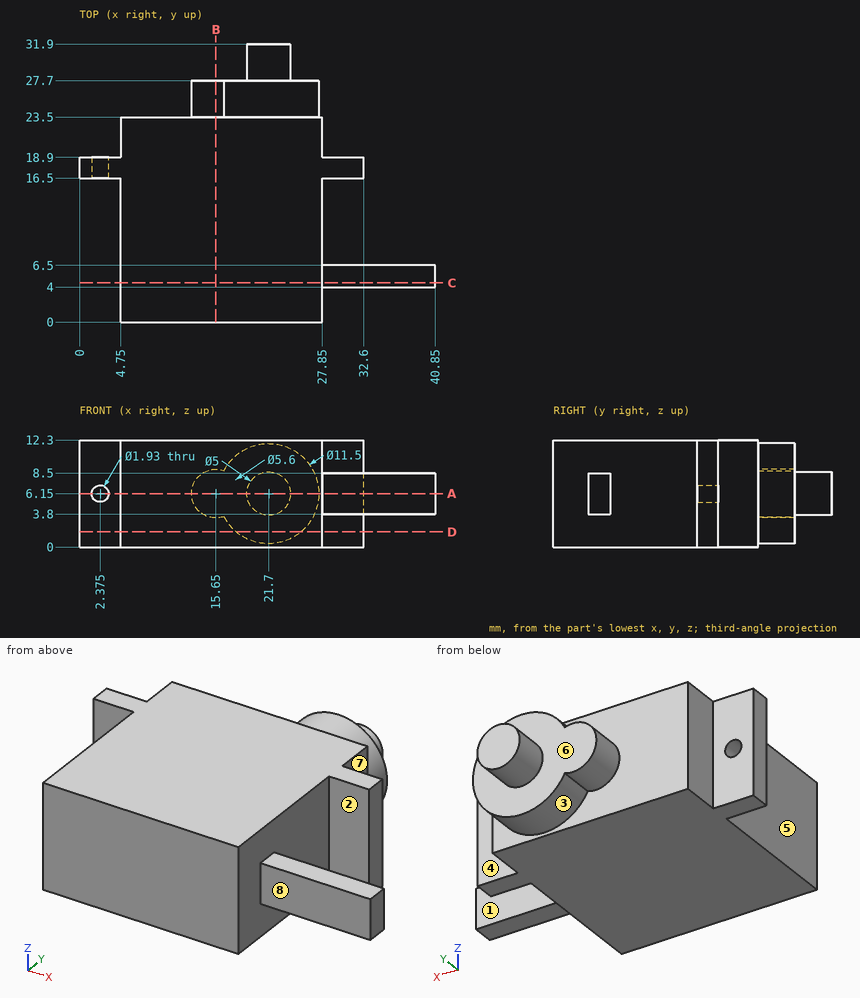
Print and shaded views of the part. All mm, measured from the part's lowest x, y and z. A direction names the side the tool comes from. Round coordinates to 2 decimals unless told otherwise and drop trailing zeros. Loops run counter-clockwise (first coordinate to the right, second up) from the corner with the lowest first, then second, coordinate; pieces in that order, holes last. Notation, with made-up numbers: M 44.25,-25.5 L 70.25,-25.5 A22 cw 70.25,2.5 Z; hole C 74,29 d7. An arc over 180 degrees is marked long. One line per question, with ' | ' between items.
1) Band-saw the part on C-C (y = 4.5). Give the cut face in (x, z), then the cut area to 3 significant figures.
Solved:
outline: M 4.75,0 L 27.85,0 L 27.85,3.8 L 40.85,3.8 L 40.85,8.5 L 27.85,8.5 L 27.85,12.3 L 4.75,12.3 Z | area: 345 mm²
2) Band-saw the part on B-B (x = 15.65). Give the cut face in (y, z).
Solved:
outline: M 0,0 L 23.5,0 L 23.5,3.35 L 27.7,3.35 L 27.7,8.95 L 23.5,8.95 L 23.5,12.3 L 0,12.3 Z
3) 3-axis set-ups, long thin cutter, end or side, ignore diameter. For the marked faces 5, 6, 7 and 8: which of +Z, -Z, +X, -X, +Y, -Y reach the whole face in a straight line?
Solved:
face 5: +Z, -Z, -X, -Y | face 6: +Y | face 7: +Z, -Z, +X, +Y | face 8: +Z, -Z, +X, -Y
4) Mould opens along Y. For the marked faces 1, 2, 3 and 4 say: +Y half, -Y half, draft (parallel to the pull), parting line (faces both ways), or undercut.
Solved:
face 1: undercut | face 2: undercut | face 3: draft | face 4: +Y half
5) Flat gauge pins, fed straight in: pin 1 (2 mm diameter, centred on x = 2.375, z = 6.15, fed in from +Y); pin 2 (1.4 mm diameter, centred on x = 29.5, z = 9, fed in from -Y); pin 3 (6 mm diameter, centred on y = 11.5, z = 5.5, fed in from -X). Where does each tip first touch, or does it go through?
Solved:
pin 1: stops at y = 18.9 | pin 2: stops at y = 4 | pin 3: stops at x = 4.75
6) Drill centre lines: line 1 along Y through (x, z) = (32, 4.25); line 2 along Y through (x, z) = (4.5, 5.5); line 3 along Y through (x, z) = (12, 8.5). Where is each one in solid material? Low to high.
Solved:
line 1: y = 4 to 6.5, 16.5 to 18.9 | line 2: y = 16.5 to 18.9 | line 3: y = 0 to 23.5
7) Band-saw the part on A-A (z = 6.15). Give the cut face in (x, y), then the cut area to 3 significant figures.
Solved:
outline: M 0,16.5 L 1.41,16.5 L 1.41,18.9 L 0,18.9 Z; M 3.34,16.5 L 4.75,16.5 L 4.75,0 L 27.85,0 L 27.85,4 L 40.85,4 L 40.85,6.5 L 27.85,6.5 L 27.85,16.5 L 32.6,16.5 L 32.6,18.9 L 27.85,18.9 L 27.85,23.5 L 27.45,23.5 L 27.45,27.7 L 24.2,27.7 L 24.2,31.9 L 19.2,31.9 L 19.2,27.7 L 12.85,27.7 L 12.85,23.5 L 4.75,23.5 L 4.75,18.9 L 3.34,18.9 Z | area: 676 mm²
8) Band-saw the part on D-D (z = 1.75). Give the cut face in (x, y), then the cut area to 3 significant figures.
Solved:
outline: M 0,16.5 L 4.75,16.5 L 4.75,0 L 27.85,0 L 27.85,16.5 L 32.6,16.5 L 32.6,18.9 L 27.85,18.9 L 27.85,23.5 L 25.4,23.5 L 25.4,27.7 L 18,27.7 L 18,23.5 L 4.75,23.5 L 4.75,18.9 L 0,18.9 Z | area: 597 mm²
